The listing builds one solid part. Answer for the finished solid, in the listing's coordinates (mm). Face numbers are marked on the shaded views. A direction names the side the tool comes from. Round coordinates to 2 decimals unless told otherwise and drop trailing zeros. Order: outer loops, then holes, each group sorted by start corner. A loop starts at its lowest first (then second) coordinate and runs counter-clockwise, first axis right, second up. Notation, with made-up numbers: (-29, 84) - (-13, 84) arc R9 ccw to (-13, 88) - close; hole circle Ø8 at (0.25, 42.25). An arc over 180 degrees is marked (long way). Write item = value, one per line.
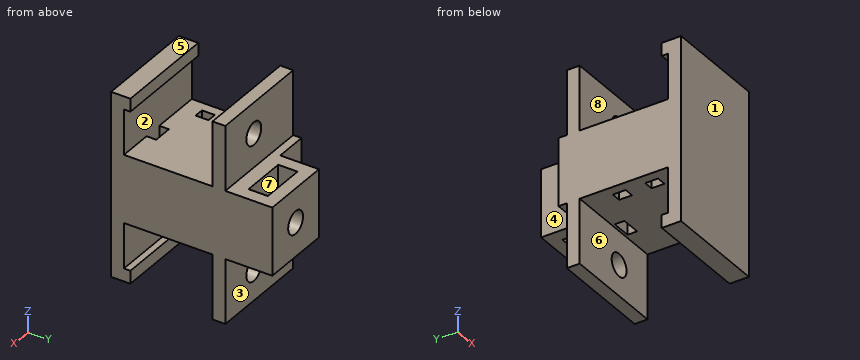
from build123d import *

# Parameters (mm, degrees)
SKETCH1_W           = 16
SKETCH1_H           = 10.5
BOSS_EXTRUDE1_DEPTH = 25
SKETCH3_W           = 16
SKETCH3_H           = 2
BOSS_EXTRUDE2_DEPTH = 7
BOSS_EXTRUDE5_START = -10.5
SKETCH3_2_W         = 16
SKETCH3_2_H         = 2
BOSS_EXTRUDE5_DEPTH = 7
SKETCH2_W           = 3
SKETCH2_H           = 1.5
SKETCH2_W_2         = 1.5
SKETCH2_H_2         = 2
CUT_EXTRUDE1_DEPTH  = 20
SKETCH5_W           = 16
SKETCH5_H           = 2
BOSS_EXTRUDE3_DEPTH = 3
BOSS_EXTRUDE6_START = -24.5
SKETCH5_2_W         = 16
SKETCH5_2_H         = 2
BOSS_EXTRUDE6_DEPTH = 3
SKETCH4_R           = 1.75
CUT_EXTRUDE2_DEPTH  = 10
SKETCH6_W           = 16
SKETCH6_H           = 3
BOSS_EXTRUDE4_DEPTH = 2
BOSS_EXTRUDE7_START = -24.5
SKETCH6_2_W         = 16
SKETCH6_2_H         = 3
BOSS_EXTRUDE7_DEPTH = 2
SKETCH7_W           = 10.5
SKETCH7_H           = 6
CUT_EXTRUDE3_DEPTH  = 5
SKETCH8_R           = 1.75
CUT_EXTRUDE4_DEPTH  = 5
SKETCH10_W          = 7
SKETCH10_H          = 3
CUT_EXTRUDE5_DEPTH  = 15


with BuildPart() as part:
    # Sketch1 → Boss-Extrude1 (new body)
    with BuildSketch(Plane(origin=(0, 0, 0), x_dir=(1, 0, 0), z_dir=(0, 1, 0))):
        with Locations((8, 5.25)):
            Rectangle(SKETCH1_W, SKETCH1_H)
    extrude(amount=BOSS_EXTRUDE1_DEPTH)

    # Sketch3 → Boss-Extrude2 (add)
    with BuildSketch(Plane.XY):
        with Locations((8, 1)):
            Rectangle(SKETCH3_W, SKETCH3_H)
        with Locations((8, 16.721705876)):
            Rectangle(SKETCH3_W, SKETCH3_H)
    extrude(amount=BOSS_EXTRUDE2_DEPTH)

    # Sketch3<2> → Boss-Extrude5 (add)
    with BuildSketch(Plane.XY.offset(BOSS_EXTRUDE5_START)):
        with Locations((8, 1)):
            Rectangle(SKETCH3_2_W, SKETCH3_2_H)
        with Locations((8, 16.721705876)):
            Rectangle(SKETCH3_2_W, SKETCH3_2_H)
    extrude(amount=-BOSS_EXTRUDE5_DEPTH)

    # Sketch2 → Cut-Extrude1 (cut)
    with BuildSketch(Plane.XY):
        with Locations((9.168058596, 2.75)):
            Rectangle(SKETCH2_W, SKETCH2_H)
        with Locations((9.127915422, 14.553433745)):
            Rectangle(SKETCH2_W, SKETCH2_H)
        with Locations((2.294862544, 5.592632304)):
            Rectangle(SKETCH2_W_2, SKETCH2_H_2)
        with Locations((2.294862544, 10.60615461)):
            Rectangle(SKETCH2_W_2, SKETCH2_H_2)
    extrude(amount=-CUT_EXTRUDE1_DEPTH, mode=Mode.SUBTRACT)

    # Sketch5 → Boss-Extrude3 (add)
    with BuildSketch(Plane.XY.offset(7)):
        with Locations((8, 16.721705876)):
            Rectangle(SKETCH5_W, SKETCH5_H)
    extrude(amount=BOSS_EXTRUDE3_DEPTH)

    # Sketch5<2> → Boss-Extrude6 (add)
    with BuildSketch(Plane.XY.offset(7).offset(BOSS_EXTRUDE6_START)):
        with Locations((8, 16.721705876)):
            Rectangle(SKETCH5_2_W, SKETCH5_2_H)
    extrude(amount=-BOSS_EXTRUDE6_DEPTH)

    # Sketch4 → Cut-Extrude2 (cut)
    with BuildSketch(Plane(origin=(0, 17.721705876, 0), x_dir=(1, 0, 0), z_dir=(0, 1, 0))):
        with Locations(Location((9.291269906, -5.227094259, 0), (0, 0, 270))):
            Circle(SKETCH4_R)
        with Locations(Location((9.291269906, 15.727094259, 0), (0, 0, 90))):
            Circle(SKETCH4_R)
    extrude(amount=-CUT_EXTRUDE2_DEPTH, mode=Mode.SUBTRACT)

    # Sketch6 → Boss-Extrude4 (add)
    with BuildSketch(Plane.XY.offset(7)):
        with Locations((8, 1.5)):
            Rectangle(SKETCH6_W, SKETCH6_H)
    extrude(amount=BOSS_EXTRUDE4_DEPTH)

    # Sketch6<2> → Boss-Extrude7 (add)
    with BuildSketch(Plane.XY.offset(7).offset(BOSS_EXTRUDE7_START)):
        with Locations((8, 1.5)):
            Rectangle(SKETCH6_2_W, SKETCH6_2_H)
    extrude(amount=-BOSS_EXTRUDE7_DEPTH)

    # Sketch7 → Cut-Extrude3 (cut)
    with BuildSketch(Plane.ZY):
        with Locations((-5.25, 22)):
            Rectangle(SKETCH7_W, SKETCH7_H)
    extrude(amount=-CUT_EXTRUDE3_DEPTH, mode=Mode.SUBTRACT)

    # Sketch8 → Cut-Extrude4 (cut)
    with BuildSketch(Plane(origin=(0, 25, 0), x_dir=(1, 0, 0), z_dir=(0, 1, 0))):
        with Locations(Location((10.5, 5.25, 0), (0, 0, 270))):
            Circle(SKETCH8_R)
    extrude(amount=-CUT_EXTRUDE4_DEPTH, mode=Mode.SUBTRACT)

    # Sketch10 → Cut-Extrude5 (cut)
    with BuildSketch(Plane.XY):
        with Locations((10.5, 21.5)):
            Rectangle(SKETCH10_W, SKETCH10_H)
    extrude(amount=-CUT_EXTRUDE5_DEPTH, mode=Mode.SUBTRACT)


solid = part.part
Q1. Section C-C on z = -12.5 is taken. Determine the outline of the cut face in (x, y), then the cut area to 3 significant figures.
Model answer:
outline = (0, 0) - (16, 0) - (16, 2) - (0, 2) - close; (0, 15.72) - (16, 15.72) - (16, 17.72) - (0, 17.72) - close
area = 64.0 mm^2
Q2. Find the intervals of material crossed by line 1 (Y direction, x = 9.75, z = -3.5); line 2 (Y direction, x = 1, z = 7.5); line 3 (X direction, y = 15, z = -1.5), in increasing order. Write a range as from..to.
Model answer:
line_1 = 0..2, 3.5..13.8, 15.3..20, 23..25
line_2 = 0..3, 15.72..17.72
line_3 = 0..7.63, 10.63..16
Q3. Section B-B on z = -5.25 is taken. Count the separate pieces of the cut face and the enclosed holes in it, then the cut area to 3 significant figures.
Model answer:
separate_pieces = 1
enclosed_holes = 4
area = 327 mm^2
Q4. For the marked faces 5, 6, 7 and 8, determine the directions among +Z, -Z, +X, -X, +Y, -Y from which every point of the face is accessible in a straight line to the end or side of a thin tool.
Model answer:
face_5 = +Z, +X, -X, -Y
face_6 = -Z, +X, -X
face_7 = +Z, -Z
face_8 = +Z, +X, -X
Q5. Flat-ended cylindrical pins translate along their axes: P1, Ø7.5, axis at x = 9, z = -5, coming from the +Y side; P2, Ø6, axis at x = 11.5, y = 23, coming from the -Z side; P3, Ø8, axis at x = 9.5, z = 4.5, coming from the +Y side; P4, Ø2.5, axis at x = 2, z = -3, coming from the +Y side. Find the tip coordinate at first contact, or state that the pin passes through.
Model answer:
P1 = 25
P2 = -10.5
P3 = 17.72
P4 = 19
Q6. Determine the mould class of the marked faces 1, 2, 3 and 4 for opening direction Y: released by +Y, released by -Y, zero draft, split by the parting line, or undercut.
Model answer:
face_1 = released by -Y
face_2 = undercut
face_3 = released by +Y
face_4 = zero draft
Q7. Section A-A on y = 14.5 is taken. Determine the outline of the cut face in (x, z), then the cut area to 4 significant figures.
Model answer:
outline = (0, -10.5) - (7.63, -10.5) - (7.63, 0) - (0, 0) - close; (10.63, -10.5) - (16, -10.5) - (16, 0) - (10.63, 0) - close
area = 136.5 mm^2
Q8. Section D-D on z = 5.5 is taken. Determine the outline of the cut face in (x, y), then the cut area to 3 significant figures.
Model answer:
outline = (0, 0) - (16, 0) - (16, 2) - (0, 2) - close; (0, 15.72) - (7.56, 15.72) - (7.56, 17.72) - (0, 17.72) - close; (11.02, 15.72) - (16, 15.72) - (16, 17.72) - (11.02, 17.72) - close
area = 57.1 mm^2
